```python
from build123d import *

# Parameters (mm, degrees)
EXTRUDE_THIN1_DEPTH = 7.62
CHAMFER1_SIZE       = 1.190625
CUT_EXTRUDE1_DEPTH  = 15.472853006
CRVPATTERN1_DEPTH   = 7.62


# Read off the part's stored shape, not the designer's step: CrvPattern1
with BuildPart() as part:
    # Sketch2 → Extrude-Thin1 (new body)
    with BuildSketch(Plane.XY):
        with BuildLine():
            Line((0, 0), (0, 10.606813737))
            ThreePointArc((0, 10.606813737), (-0.463285182, 11.191030357), (-1.137696862, 10.873050632))
            Line((-1.137696862, 10.873050632), (-4.664645747, 3.749960706))
            ThreePointArc((-4.664645747, 3.749960706), (-5.08, 1.975048069), (-4.664645747, 0.200135433))
            Line((-4.664645747, 0.200135433), (-3.82620918, -1.493186263))
            Line((-3.82620918, -1.493186263), (-3.553059174, -1.35793792))
            Line((-3.553059174, -1.35793792), (-4.391495741, 0.335383776))
            ThreePointArc((-4.391495741, 0.335383776), (-4.7752, 1.975048069), (-4.391495741, 3.614712363))
            Line((-4.391495741, 3.614712363), (-0.864546856, 10.737802289))
            ThreePointArc((-0.864546856, 10.737802289), (-0.53273631, 10.894248314), (-0.3048, 10.606813737))
            Line((-0.3048, 10.606813737), (-0.3048, 0))
            Line((-0.3048, 0), (0, 0))
        make_face()
    extrude(amount=EXTRUDE_THIN1_DEPTH)

    # Chamfer1
    chamfer1_edges = [part.edges().sort_by_distance(p)[0] for p in [
        (-3.689634177, -1.425562092, 0),
        (-3.689634177, -1.425562092, 7.62),
    ]]
    chamfer(chamfer1_edges, length=CHAMFER1_SIZE)

    # Sketch4 → Cut-Extrude1 (cut, through all)
    with BuildSketch(Plane.XY.offset(7.62)):
        with BuildLine():
            Line((-4.664645747, 3.749960706), (-4.596046712, 3.664267155))
            Line((-4.596046712, 3.664267155), (-4.705815616, 3.664267155))
            ThreePointArc((-4.705815616, 3.664267155), (-4.685485281, 3.707236248), (-4.664645747, 3.749960706))
        make_face()
    extrude(amount=-CUT_EXTRUDE1_DEPTH, mode=Mode.SUBTRACT)

    # CrvPattern1 outline → CrvPattern1 (cut)
    with BuildSketch(Plane.XY):
        with BuildLine():
            Line((-4.744975764, 0.372564793), (-4.680378039, 0.445121042))
            Line((-4.680378039, 0.445121042), (-4.777966042, 0.450237541))
            ThreePointArc((-4.777966042, 0.450237541), (-4.761675743, 0.411314165), (-4.744975764, 0.372564793))
        make_face()
        with BuildLine():
            ThreePointArc((-4.748910862, 3.568501265), (-4.767580416, 3.524806333), (-4.785729607, 3.48089271))
            Line((-4.785729607, 3.48089271), (-4.676162545, 3.486332727))
            Line((-4.676162545, 3.486332727), (-4.748910862, 3.568501265))
        make_face()
        with BuildLine():
            ThreePointArc((-4.824009644, 3.383022425), (-4.840450562, 3.338503815), (-4.856362147, 3.293793281))
            Line((-4.856362147, 3.293793281), (-4.747356217, 3.304644344))
            Line((-4.747356217, 3.304644344), (-4.824009644, 3.383022425))
        make_face()
        with BuildLine():
            ThreePointArc((-4.889747992, 3.19399033), (-4.903912846, 3.148798701), (-4.917541653, 3.103442532))
            Line((-4.917541653, 3.103442532), (-4.809452549, 3.119649065))
            Line((-4.809452549, 3.119649065), (-4.889747992, 3.19399033))
        make_face()
        with BuildLine():
            ThreePointArc((-4.945955852, 3.001880747), (-4.957808713, 2.956169664), (-4.969121106, 2.910321838))
            Line((-4.969121106, 2.910321838), (-4.862298748, 2.931802088))
            Line((-4.862298748, 2.931802088), (-4.945955852, 3.001880747))
        make_face()
        with BuildLine():
            ThreePointArc((-4.992487715, 2.807177794), (-5.002004339, 2.761102753), (-5.010978384, 2.714918968))
            Line((-5.010978384, 2.714918968), (-4.905764782, 2.741565627))
            Line((-4.905764782, 2.741565627), (-4.992487715, 2.807177794))
        make_face()
        with BuildLine():
            ThreePointArc((-5.02922305, 2.610372633), (-5.036390971, 2.564090075), (-5.043016507, 2.517726765))
            Line((-5.043016507, 2.517726765), (-4.939743698, 2.549407773))
            Line((-4.939743698, 2.549407773), (-5.02922305, 2.610372633))
        make_face()
        with BuildLine():
            ThreePointArc((-5.056066661, 2.411962141), (-5.060885198, 2.365628463), (-5.06516382, 2.319241812))
            Line((-5.06516382, 2.319241812), (-4.96415189, 2.355801348))
            Line((-4.96415189, 2.355801348), (-5.056066661, 2.411962141))
        make_face()
        with BuildLine():
            ThreePointArc((-5.07294897, 2.212447566), (-5.075429139, 2.166218137), (-5.077374093, 2.1199631))
            Line((-5.077374093, 2.1199631), (-4.978929297, 2.161222738))
            Line((-4.978929297, 2.161222738), (-5.07294897, 2.212447566))
        make_face()
        with BuildLine():
            ThreePointArc((-5.079826224, 2.012333162), (-5.079990568, 1.966361356), (-5.079626554, 1.920390698))
            Line((-5.079626554, 1.920390698), (-4.98403956, 1.966150718))
            Line((-4.98403956, 1.966150718), (-5.079826224, 2.012333162))
        make_face()
        with BuildLine():
            ThreePointArc((-5.076680625, 1.812124816), (-5.074562951, 1.766561064), (-5.071925849, 1.721024422))
            Line((-5.071925849, 1.721024422), (-4.979470103, 1.771065282))
            Line((-4.979470103, 1.771065282), (-5.076680625, 1.812124816))
        make_face()
        with BuildLine():
            ThreePointArc((-5.063520382, 1.612328668), (-5.059165421, 1.567319544), (-5.054301926, 1.522362527))
            Line((-5.054301926, 1.522362527), (-4.965232171, 1.576446452))
            Line((-4.965232171, 1.576446452), (-5.063520382, 1.612328668))
        make_face()
        with BuildLine():
            ThreePointArc((-5.040379693, 1.413449735), (-5.033842672, 1.369137078), (-5.026809852, 1.324900401))
            Line((-5.026809852, 1.324900401), (-4.941360798, 1.382773106))
            Line((-4.941360798, 1.382773106), (-5.040379693, 1.413449735))
        make_face()
        with BuildLine():
            ThreePointArc((-5.007318634, 1.215990531), (-4.998664778, 1.172510618), (-4.989529564, 1.129129286))
            Line((-4.989529564, 1.129129286), (-4.907914719, 1.190521793))
            Line((-4.907914719, 1.190521793), (-5.007318634, 1.215990531))
        make_face()
        with BuildLine():
            ThreePointArc((-4.964422988, 1.020449699), (-4.953726948, 0.977932464), (-4.942565548, 0.935535016))
            Line((-4.942565548, 0.935535016), (-4.864976234, 1.000165564))
            Line((-4.864976234, 1.000165564), (-4.964422988, 1.020449699))
        make_face()
        with BuildLine():
            ThreePointArc((-4.911803987, 0.827320662), (-4.899149207, 0.785888981), (-4.886046457, 0.744596783))
            Line((-4.886046457, 0.744596783), (-4.812650995, 0.812172807))
            Line((-4.812650995, 0.812172807), (-4.911803987, 0.827320662))
        make_face()
        with BuildLine():
            ThreePointArc((-4.849597983, 0.63709028), (-4.835076, 0.596859317), (-4.820124666, 0.556785934))
            Line((-4.820124666, 0.556785934), (-4.751067753, 0.627006093))
            Line((-4.751067753, 0.627006093), (-4.849597983, 0.63709028))
        make_face()
    extrude(amount=CRVPATTERN1_DEPTH, mode=Mode.SUBTRACT)


solid = part.part
```
Source: CAD feature listing. Evaluate the final solid. Frame: model axes, mm. A direction names the side the tool comes from. Round coordinates to 2 decimals unless told otherwise and drop trailing zeros. Order: outer loops, then holes, each group sorted by start corner. A loop starts at its lowest first (then second) coordinate and runs counter-clockwise, first axis right, second up. Notation, with made-up numbers: (9.5, -3) -> (17.5, -3) arc R21 ccw to (17.5, 28) -> close; hole circle Ø1 at (77.25, 45.25). An arc over 180 degrees is marked (long way). One line per item, written item: value. Start each with the question number.
Q1. Draft query along Y for faces 1 (the flat face through (-4.251, -0.635, 3.757)), 2 (the flat face through (-2.65, 7.13, 3.76)), 3 (the flat face through (-0.305, 5, 4)), 4 (the cylindrical face through (-4.775, 1.951, 3.757)). Return one class per face: pulls with the +Y half, pulls with the -Y half, needs draft (parallel to the pull), parting line crosses it, or undercut.
Q2. Access query for faces 5 (the flat face through (-3.959, -0.886, 0.587)), 6 (the flat face through (-3.97, -0.52, 3.76)). Directions: +Z, -Z, +X, -X, +Y, -Y. A direction counts if a zero-diameter tool reaches every point of the face in a straight line with its end or side. Return the directions, or none.
Q3. Material intervals for probe 1 along X at (y, z) = (5.5, 3.5); probe 2 along X at (y, z) = (10, 5.5); probe 3 along Y at (x, z) = (-3.2, 1.25), sorted ascending.
Q4. Section query B-B (x = -1.35). Return the cut outline in (y, z).
Q5. Section query A-A (y = 4.25). Return the cut outline in (x, z).
Q6. Pin query (flat end, axial travel): pin 1 (2 mm diameter, centred on x = -4.5, z = 1, fed in from +Y); pin 2 (1.5 mm diameter, centred on x = -4, z = 4.5, fed in from +Y). Return the tip coordinate at first contact, or that it passes through.
Findings below:
1. face 1: pulls with the -Y half
1. face 2: undercut
1. face 3: needs draft
1. face 4: undercut
2. face 5: -Z, +X, -Y
2. face 6: +Z, -Z
3. probe 1: -3.8 to -3.46, -0.3 to 0
3. probe 2: -1.57 to -1.23, -0.3 to 0
3. probe 3: 6.02 to 6.71
4. outline: (9.76, 0) -> (10.44, 0) -> (10.44, 7.62) -> (9.76, 7.62) -> close
5. outline: (-4.42, 0) -> (-4.08, 0) -> (-4.08, 7.62) -> (-4.42, 7.62) -> close; (-0.3, 0) -> (0, 0) -> (0, 7.62) -> (-0.3, 7.62) -> close
6. pin 1: y = 6.1
6. pin 2: y = 6.61
